The model under review builds one solid part; all positions refer to its coordinate system, in mm. A direction names the side the tool comes from. Round coordinates to 2 decimals unless told otherwise and drop trailing zeros. Write each loop counter-clockwise with the first axis right and the second up, starting at its lowest first coordinate (ties: lowest second). Pieces come first, ordered by that corner, then holes. Notation, with made-up numbers: (2.5, -31.75) -> (42.5, -31.75) arc R14 ccw to (42.5, -4.75) -> close; hole circle Ø8 at (35, -20.75). An arc over 180 degrees is marked (long way). Answer as a JSON object with one key per item and string values. Group by question number.
1) To check wall thickness, follow probe 1 along Z at (x, y) = (9.5, -5); probe 2 along Z at (x, y) = (15.25, 1.25); probe 3 along Y at (x, z) = (13.75, 5.75). State the ranges of each line that lie inside material, in increasing order. Write a range as [from, to].
2) Insertion check: pin 1 Ø14 at (y, z) = (0, 0) entering from +X; pin 2 Ø1 at (x, y) = (3.5, -9) entering from -Z; pin 3 Ø1 at (y, z) = (8.5, -7.5) entering from -X. Each pin has a flat end and moves straight along its axis. Give the tip position at first contact, or say it passes through.
3) We need section A-A, the plane x = 5.75. Write out the cut boundary in (y, z), then the cut area to 3 significant figures.
4) Mouldability with a two-part tool opening along Y and no side actions: class faces 4 (the flat face through (10, 0, 12)), 5 (the cylindrical face through (3.976, -5.786, 5.305)), 6 (the cylindrical face through (10.577, 6.585, -11.44)), 7 (the conical face through (4.297, -12.362, 0.079)) as pulls with the +Y half, pulls with the -Y half, needs draft (parallel to the pull), parting line crosses it, or undercut.
5) We need section B-B, the plane x = 9.5. Write out the cut boundary in (y, z).
6) Machinability: for faces 1 (the conical face through (11.17, 8.916, 2.808)), 2 (the flat face through (9.911, 10.431, 5.933)), 3 (the cylindrical face through (5.857, -2.027, -9.128)), which of the approach directions +Z, -Z, +X, -X, +Y, -Y give a long, thin tool a straight path to every point of the face, cutting with its end or side? Answer none if there is none.
7) We need section C-C, the plane x = 2. Write out the cut boundary in (y, z), then the cut area to 3 significant figures.
Autodesk Inventor part; units mm, degrees
ref_plane "IP1_XY" through (0, 0, 0) normal (1, 0, 0) x (0, 0, -1)
ref_plane "IP1_YZ" through (0, 0, 0) normal (0, 0, -1) x (0, 1, 0)
ref_plane "IP1_ZX" through (0, 0, 0) normal (0, 1, 0) x (1, 0, 0)
sketch "Sketch_1" plane through (0, 0, 0) normal (0, 0, 1) x (1, 0, 0)
  line L0 (16, 0) -> (0, 0)
  line L1 (0, 0) -> (0, 8.35)
  arc A0 (3.5, 11.85) -> (0, 8.35) centre (3.5, 8.35) ccw
  line L2 (3.5, 11.85) -> (3.6341, 11.85)
  arc A1 (3.6341, 11.85) -> (4.0171, 12.0286) centre (3.6341, 12.35) ccw
  line L3 (4.0171, 12.0286) -> (5, 13.2)
  line L4 (5, 13.2) -> (16, 13.2)
  line L5 (16, 13.2) -> (16, 0)
  line L6 (16, 0) -> (0, 0)
revolve "Revolution1" add sketch "Sketch_1" angle 360 about axis through (16, 0, 0) along (1, 0, 0)
sketch "Sketch_2" plane through (0, 0, 0) normal (1, 0, 0) x (0, 1, 0)
  line L0 (-24, 24) -> (-24, -24)
  line L1 (-24, -24) -> (24, -24)
  line L2 (24, -24) -> (24, 24)
  line L3 (24, 24) -> (-24, 24)
  line L4 (-6.9282, 12) -> (-13.8564, 0)
  line L5 (-13.8564, 0) -> (-6.9282, -12)
  line L6 (-6.9282, -12) -> (6.9282, -12)
  line L7 (6.9282, -12) -> (13.8564, 0)
  line L8 (13.8564, 0) -> (6.9282, 12)
  line L9 (6.9282, 12) -> (-6.9282, 12)
extrude "Extrusion1" cut sketch "Sketch_2" along normal blind 16
sketch "Sketch_3" plane through (0, 0, 0) normal (0, 0, 1) x (1, 0, 0)
  line L0 (16, 0) -> (-0.2, 0)
  line L1 (-0.2, 0) -> (-0.2, 7.05)
  line L2 (-0.2, 7.05) -> (0, 7.05)
  arc A0 (0, 7.05) -> (1, 6.05) centre (1, 7.05) ccw
  line L3 (1, 6.05) -> (2.554, 6.05)
  arc A1 (2.554, 6.05) -> (3.7, 6.6458) centre (2.554, 7.45) ccw
  line L4 (3.7, 6.6458) -> (3.7, 7.85)
  line L5 (3.7, 7.85) -> (4.2447, 7.85)
  line L6 (4.2447, 7.85) -> (4.8414, 9.2557)
  arc A2 (4.8874, 9.35) -> (4.8414, 9.2557) centre (5.7619, 8.865) ccw
  line L7 (4.8874, 9.35) -> (6.8, 9.35)
  line L8 (6.8, 9.35) -> (6.8, 9.3)
  line L9 (6.8, 9.3) -> (15.419, 9.3937)
  line L10 (15.419, 9.3937) -> (16, 10.4)
  line L11 (16, 10.4) -> (16, 0)
  line L12 (16, 0) -> (-0.2, 0)
revolve "Revolution2" cut sketch "Sketch_3" angle 360 about axis through (16, 0, 0) along (1, 0, 0)
ref_plane "IP1_XY" through (0, 0, 0) normal (1, 0, 0) x (0, 0, -1)
ref_plane "IP1_YZ" through (0, 0, 0) normal (0, 0, -1) x (0, 1, 0)
ref_plane "IP1_ZX" through (0, 0, 0) normal (0, 1, 0) x (1, 0, 0)
properties part number "HSK-K 1.209.1201.70-Nut"
Here are the results:
{
 "1": {"probe 1": "z = [-12, -7.88], [7.88, 12]", "probe 2": "z = [-12, -9.31], [9.31, 12]", "probe 3": "y = [-10.54, -7.41], [7.41, 10.54]"},
 "2": {"pin 1": "stops at x = 3.7", "pin 2": "stops at z = -8.26", "pin 3": "stops at x = 1.04"},
 "3": {"outline": "(-13.14, -1.24) -> (-7.64, -10.76) arc R13.2 ccw to (-5.5, -12) -> (5.5, -12) arc R13.2 ccw to (7.64, -10.76) -> (13.14, -1.24) arc R13.2 ccw to (13.14, 1.24) -> (7.64, 10.76) arc R13.2 ccw to (5.5, 12) -> (-5.5, 12) arc R13.2 ccw to (-7.64, 10.76) -> (-13.14, 1.24) arc R13.2 ccw to start; hole circle Ø18.7 at (0, 0)", "area": "219 mm^2"},
 "4": {"face 4": "needs draft", "face 5": "undercut", "face 6": "pulls with the +Y half", "face 7": "pulls with the -Y half"},
 "5": {"outline": "(-13.14, -1.24) -> (-7.64, -10.76) arc R13.2 ccw to (-5.5, -12) -> (5.5, -12) arc R13.2 ccw to (7.64, -10.76) -> (13.14, -1.24) arc R13.2 ccw to (13.14, 1.24) -> (7.64, 10.76) arc R13.2 ccw to (5.5, 12) -> (-5.5, 12) arc R13.2 ccw to (-7.64, 10.76) -> (-13.14, 1.24) arc R13.2 ccw to start; hole circle Ø18.66 at (0, 0)"},
 "6": {"face 1": "+X", "face 2": "+Z, +X, -X, +Y", "face 3": "none"},
 "7": {"outline": "circle Ø23.02 at (0, 0); hole circle Ø12.1 at (0, 0)", "area": "301 mm^2"}
}
